For this review, take the finished solid that the model builds, in its own axes (mm). A direction names the side the tool comes from. Coordinates: 2 decimals unless noted, no trailing zeros. Write each loop counter-clockwise with the first axis right and the second up, starting at its lowest first coordinate (ties: lowest second). Pieces come first, ordered by that corner, then holes. Notation, with made-up numbers: (-26, 66.5) -> (13, 66.5) arc R4 ccw to (13, 73.5) -> close; hole circle Ø8 at (48.25, 68.5). An arc over 180 degrees is marked (long way). Put each result on its own line as item: value. Start each with the question number.
Item 1: The part is to be moulded in two halves that separate along X. For faces 1 (the flat face through (47.225, -24.124, 2.465)), 2 (the flat face through (52, -30, 2)), 3 (the flat face through (49, -32.495, 2)), say which applies: +X half, -X half, draft (parallel to the pull), parting line (faces both ways), or undercut.
Item 2: Consider section B-B on x = 36. Give the boundary of the cut face in (y, z), and give its area (3 significant figures).
Item 3: Consider section A-A on z = 1.1. Give the boundary of the cut face in (x, y).
Item 4: To check wall thickness, follow L1, parallel to X at y = 2, z = 3.85; L2, parallel to X at y = -7, z = 1.35; L3, parallel to Y at x = 26.5, z = 4. State the ranges of each line that lie inside material, in increasing order.
Item 5: Insertion check: P1, Ø3, axis at y = -14, z = 3.5, coming from the -X side; P2, Ø1.3, axis at x = 37, z = 1.5, coming from the +Y side; P3, Ø2, axis at y = -7, z = 2, coming from the +X side. Each pin has a flat end and moves straight along its axis. Give the tip position at first contact, or say it passes through.
Item 6: For faces 4 (the flat face through (4.95, 2, 2)), 5 (the flat face through (37, 0, 2)), 6 (the flat face through (0, -2, 2)), list the 3-axis set-ups (+Z, -Z, +X, -X, +Y, -Y) from which the entire face can be reached by the end or side of a thin tool; tool diameter is ignored.
Item 7: Consider section C-C on y = -6. Give the boundary of the cut face in (x, z), and give its area (3 significant figures).
```python
from build123d import *

# Parameters (mm, degrees)
BOSS_EXTRUDE1_DEPTH = 5
FILLET1_R           = 1


with BuildPart() as part:
    # Sketch1 → Boss-Extrude1 (new body)
    with BuildSketch(Plane.XY):
        Polygon((42, -4.582575695), (37.417424305, -6.582575695), (45.417424305, -24.912878475), (50, -22.912878475), (52, -27.49545417), (52, -32.49545417), (47, -32.49545417), (0, -5), (0, 0), (4.95, 0), (4.95, 5), (35.05, 5), (35.05, 0), (40, 0), align=None)
    extrude(amount=BOSS_EXTRUDE1_DEPTH)

    # Fillet1
    fillet1_edges = [part.edges().sort_by_distance(p)[0] for p in [
        (4.95, 5, 2.5),
        (35.05, 5, 2.5),
        (40, 0, 2.5),
        (42, -4.582575695, 2.5),
        (50, -22.912878475, 2.5),
        (52, -27.49545417, 2.5),
        (52, -32.49545417, 2.5),
        (47, -32.49545417, 2.5),
        (0, -5, 2.5),
    ]]
    fillet(fillet1_edges, radius=FILLET1_R)


solid = part.part
```
Return value:
1. face 1: undercut
1. face 2: +X half
1. face 3: draft
2. outline: (-26.06, 0) -> (0, 0) -> (0, 5) -> (-26.06, 5) -> close
2. area: 130 mm^2
3. outline: (0, -4.43) arc R1 ccw to (0.5, -5.29) -> (46.77, -32.36) arc R1 ccw to (47.27, -32.5) -> (51, -32.5) arc R1 ccw to (52, -31.5) -> (52, -27.7) arc R1 ccw to (51.92, -27.3) -> (50.4, -23.83) arc R1 ccw to (49.08, -23.31) -> (45.42, -24.91) -> (37.42, -6.58) -> (41.08, -4.98) arc R1 ccw to (41.6, -3.67) -> (40.26, -0.6) arc R1 ccw to (39.35, 0) -> (35.05, 0) -> (35.05, 4) arc R1 ccw to (34.05, 5) -> (5.95, 5) arc R1 ccw to (4.95, 4) -> (4.95, 0) -> (0, 0) -> close
4. L1: 4.95 to 35.05
4. L2: 3.42 to 37.6
4. L3: -20.5 to 5
5. P1: x = 12.82
5. P2: y = 0
5. P3: x = 38.75
6. face 4: +Z, -Z, -X, +Y
6. face 5: +Z, -Z, +X, +Y
6. face 6: +Z, -Z, -X, +Y, -Y
7. outline: (1.71, 0) -> (38.75, 0) -> (38.75, 5) -> (1.71, 5) -> close
7. area: 185 mm^2
